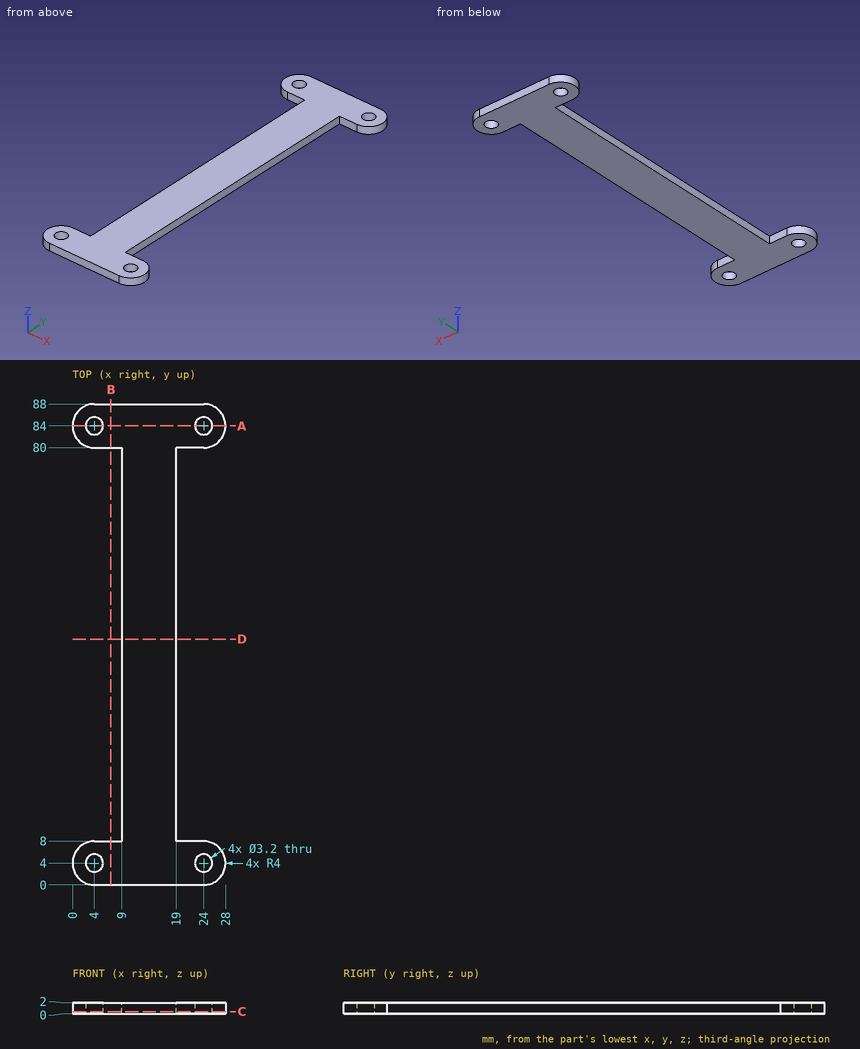
Source: three-view drawing plus pictorial views. Frame: mm from the lowest corner of the part. Round coordinates to 2 decimals unless told otherwise and drop trailing zeros. Loops run counter-clockwise (first coordinate to the right, second up) from the corner with the lowest first, then second, coordinate; pieces in that order, holes last.
Q1. Section C-C, the plane z = 0.4. Return loops of the section in (x, y).
Q2. Section B-B, the plane x = 7. Return loops of the section in (y, z), plus the area to 3 significant figures.
Q3. Ray query, line 1 (Y direction, x = 24, z = 1.1); line 2 (X direction, y = 84, z = 0.5); line 3 (Y direction, x = 20, z = 1.25). Return the intervals inside material, ascending.
Q4. Section D-D, the plane y = 45. Return loops of the section in (x, z).
Q5. Section A-A, the plane y = 84. Return loops of the section in (x, z).
Solutions:
1. outline: (4, 0) - (24, 0) arc R4 ccw to (24, 8) - (19, 8) - (19, 80) - (24, 80) arc R4 ccw to (24, 88) - (4, 88) arc R4 ccw to (4, 80) - (9, 80) - (9, 8) - (4, 8) arc R4 ccw to start; hole circle Ø3.2 at (4, 4); hole circle Ø3.2 at (4, 84); hole circle Ø3.2 at (24, 4); hole circle Ø3.2 at (24, 84)
2. outline: (0, 0) - (8, 0) - (8, 2) - (0, 2) - close; (80, 0) - (88, 0) - (88, 2) - (80, 2) - close
2. area: 32.0 mm2
3. line 1: y = 0 to 2.4, 5.6 to 8, 80 to 82.4, 85.6 to 88
3. line 2: x = 0 to 2.4, 5.6 to 22.4, 25.6 to 28
3. line 3: y = 0 to 8, 80 to 88
4. outline: (9, 0) - (19, 0) - (19, 2) - (9, 2) - close
5. outline: (0, 0) - (2.4, 0) - (2.4, 2) - (0, 2) - close; (5.6, 0) - (22.4, 0) - (22.4, 2) - (5.6, 2) - close; (25.6, 0) - (28, 0) - (28, 2) - (25.6, 2) - close
